from build123d import *

# Parameters (mm, degrees)
SKETCH1_W           = 25.4
SKETCH1_H           = 163.454078658
SKETCH1_R           = 3.175
BOSS_EXTRUDE1_DEPTH = 6.35
FILLET2_R           = 12.7
FILLET3_R           = 2.116666667


with BuildPart() as part:
    # Sketch1 → Boss-Extrude1 (new body)
    with BuildSketch(Plane(origin=(0, 0, 0), x_dir=(1, 0, 0), z_dir=(0, 1, 0))):
        Rectangle(SKETCH1_W, SKETCH1_H)
        with Locations(Location((0, -69.027039329, 0), (0, 0, 270))):
            Circle(SKETCH1_R, mode=Mode.SUBTRACT)
        with Locations(Location((0, 69.027039329, 0), (0, 0, 270))):
            Circle(SKETCH1_R, mode=Mode.SUBTRACT)
    extrude(amount=BOSS_EXTRUDE1_DEPTH)

    # Fillet2
    fillet2_edges = [part.edges().sort_by_distance(p)[0] for p in [
        (-12.7, 3.175, -81.727039329),
        (12.7, 3.175, -81.727039329),
        (-12.7, 3.175, 81.727039329),
        (12.7, 3.175, 81.727039329),
    ]]
    fillet(fillet2_edges, radius=FILLET2_R - 0.0001)  # a hair under: the kernel refuses the full size

    # Fillet3
    fillet3_edges = [part.edges().sort_by_distance(p)[0] for p in [
        (-12.7, 0, 0),
        (-12.7, 6.35, 0),
        (12.7, 0, 0),
        (8.98028541, 0, 78.007324739),
        (-8.98028541, 0, 78.007324739),
        (8.98028541, 0, -78.007324739),
        (-8.98028541, 0, -78.007324739),
        (12.7, 6.35, 0),
        (8.98028541, 6.35, 78.007324739),
        (-8.98028541, 6.35, 78.007324739),
        (8.98028541, 6.35, -78.007324739),
        (-8.98028541, 6.35, -78.007324739),
    ]]
    fillet(fillet3_edges, radius=FILLET3_R)


solid = part.part
Part model, mm, in its own coordinate system. Coordinates: 2 decimals unless noted, no trailing zeros. Order: outer loops, then holes, each group sorted by start corner. A loop starts at its lowest first (then second) coordinate and runs counter-clockwise, first axis right, second up.
(1) Slice it at B-B, the plane y = 3.25. State how many separate pieces and enclosed holes the cut face has, and give its area (3 significant figures).
Check sheet entries:
separate pieces: 1
enclosed holes: 2
area: 3,950 mm2
(2) Slice it at A-A, the plane z = 25.5. Write the cut outline in (x, y), and give its area (3 significant figures).
Check sheet entries:
outline: (-12.7, 2.12) arc R2.12 ccw to (-10.58, 0) - (10.58, 0) arc R2.12 ccw to (12.7, 2.12) - (12.7, 4.23) arc R2.12 ccw to (10.58, 6.35) - (-10.58, 6.35) arc R2.12 ccw to (-12.7, 4.23) - close
area: 157 mm2
(3) Slice it at C-C, the plane z = -67.5. Write the cut outline in (x, y).
Check sheet entries:
outline: (-12.7, 2.12) arc R2.12 ccw to (-10.58, 0) - (-2.78, 0) - (-2.78, 6.35) - (-10.58, 6.35) arc R2.12 ccw to (-12.7, 4.23) - close; (2.78, 0) - (10.58, 0) arc R2.12 ccw to (12.7, 2.12) - (12.7, 4.23) arc R2.12 ccw to (10.58, 6.35) - (2.78, 6.35) - close
(4) Pin check, flat tips, straight feed: pin 1 Ø1.5 at (x, y) = (-2, 2.5) entering from +Z; pin 2 Ø5.5 at (x, z) = (0, 69.03) entering from -Y; pin 3 Ø1 at (x, y) = (3, 1) entering from +Z; pin 4 Ø1 at (x, y) = (-9, 4.5) entering from +Z. Stop position of each tip, or through.
Check sheet entries:
pin 1: stops at z = 81.67
pin 2: passes through
pin 3: stops at z = 81.31
pin 4: stops at z = 78.45
(5) Pull direction Z, two halves, no side cores. Call faces 1 (the face through (0.954, 3.131, -65.999)), 2 (the face through (-9.078, 3.19, 77.908)), 3 (the face through (0, 6.35, -1)): pulls with the +Z half, pulls with the -Z half, needs draft (parallel to the pull), parting line crosses it, or undercut.
Check sheet entries:
face 1: undercut
face 2: pulls with the +Z half
face 3: needs draft
(6) Probe L1, parallel to Z at x = -2, y = 6; L2, parallel to Z at x = -0.75, y = 0.75; L3, parallel to X at y = 1.5, z = 71.5. List the from-to ranges inside material, lowest first.
Check sheet entries:
L1: z = -80.6 to -71.49, -66.56 to 66.56, 71.49 to 80.6
L2: z = -81.2 to -72.11, -65.94 to 65.94, 72.11 to 81.2
L3: x = -12.36 to -1.99, 1.99 to 12.36
